from build123d import *

# Parameters (mm, degrees)
SKETCH_1_R           = 14.5
EXTRUDE_1_DEPTH      = 17.3
SKETCH_2_R           = 1.475
EXTRUDE_2_DEPTH      = 8.2
MM_CLEARANCE_1_D     = 3
MM_CLEARANCE_1_DEPTH = 3
MM_CLEARANCE_1_TIP   = 0.901290929
CHAMFER_1_SIZE       = 1
CHAMFER_1_SIZE2      = 3.732050808
FILLET_1_R           = 1
CHAMFER_2_SIZE       = 1
CHAMFER_2_SIZE2      = 3.732050808
MM_CLEARANCE_2_D     = 2
MM_CLEARANCE_2_DEPTH = 3
MM_CLEARANCE_2_TIP   = 0.600860619


with BuildPart() as part:
    # 草图1 → 凸台-拉伸1 (new body)
    with BuildSketch(Plane(origin=(0, 0, 0), x_dir=(1, 0, 0), z_dir=(0, 1, 0))):
        Circle(SKETCH_1_R)
    extrude(amount=EXTRUDE_1_DEPTH)

    # 草图2 → 凸台-拉伸2 (add)
    with BuildSketch(Plane(origin=(0, 17.3, 0), x_dir=(1, 0, 0), z_dir=(0, 1, 0))):
        Circle(SKETCH_2_R)
    extrude(amount=EXTRUDE_2_DEPTH)

    # 大小mm Clearance 暗销槽口1
    with Locations(Plane(origin=(0, 0, 0), x_dir=(-1, 0, 0), z_dir=(0, -1, 0))):
        with Locations((0, -8), (9.5, 0), (0, 8.000635696), (-9.5, 0)):
            Hole(MM_CLEARANCE_1_D / 2, depth=MM_CLEARANCE_1_DEPTH)
            with Locations((0, 0, -(MM_CLEARANCE_1_DEPTH + MM_CLEARANCE_1_TIP / 2))):  # 118° drill point
                Cone(0, MM_CLEARANCE_1_D / 2, MM_CLEARANCE_1_TIP, mode=Mode.SUBTRACT)

    # 倒角1
    chamfer_1_edges = [part.edges().sort_by_distance(p)[0] for p in [
        (-14.5, 0, 0),
    ]]
    chamfer_1_side = [part.faces().sort_by_distance(p)[0] for p in [
        (0, 0, 7.107e-06),
    ]]
    chamfer(chamfer_1_edges, length=CHAMFER_1_SIZE, length2=CHAMFER_1_SIZE2, reference=chamfer_1_side[0])

    # 圆角1
    fillet_1_edges = [part.edges().sort_by_distance(p)[0] for p in [
        (-13.5, 0, 0),
    ]]
    fillet(fillet_1_edges, radius=FILLET_1_R)

    # 倒角2
    chamfer_2_edges = [part.edges().sort_by_distance(p)[0] for p in [
        (-14.5, 17.3, 0),
    ]]
    chamfer_2_side = [part.faces().sort_by_distance(p)[0] for p in [
        (-14.5, 10.516025404, 0),
    ]]
    chamfer(chamfer_2_edges, length=CHAMFER_2_SIZE, length2=CHAMFER_2_SIZE2, reference=chamfer_2_side[0])

    # 大小mm Clearance 暗销槽口2
    with Locations(Plane(origin=(0, 17.3, 0), x_dir=(1, 0, 0), z_dir=(0, 1, 0))):
        with Locations((-4.460030829, 2.575), (4.460030829, 2.575), (0, -5.15)):
            Hole(MM_CLEARANCE_2_D / 2, depth=MM_CLEARANCE_2_DEPTH)
            with Locations((0, 0, -(MM_CLEARANCE_2_DEPTH + MM_CLEARANCE_2_TIP / 2))):  # 118° drill point
                Cone(0, MM_CLEARANCE_2_D / 2, MM_CLEARANCE_2_TIP, mode=Mode.SUBTRACT)


solid = part.part
Work out the finished part from the listing and answer in its coordinate system (mm). A direction names the side the tool comes from. Give positions to 0.01 mm unless a question says otherwise; leave off trailing zeros. Write each loop counter-clockwise with the first axis right and the second up, starting at its lowest first coordinate (ties: lowest second). Pieces come first, ordered by that corner, then holes. Notation, with made-up numbers: M -37.5,84.25 L -29.5,84.25 A6 ccw -29.5,93.25 Z; hole C 55,23 d3. An arc over 180 degrees is marked long. Answer as CSV lines item,"result".
Q1. The mould has two halves that part along X. Classify faces 1 (the cylindrical face through (-1.474, 21.343, -0.065)), 2 (the flat face through (0, 17.3, 2)), 3 (the cylindrical face through (3.506, 15.779, -2.875)), 4 (the cylindrical face through (-11, 2, 0)): +X half, -X half, draft (parallel to the pull), parting line (faces both ways), or undercut.
A:
face 1,"parting line"
face 2,"draft"
face 3,"undercut"
face 4,"undercut"
Q2. A cutting plane is placed at A-A on y = 21. Write down the section's boundary in (x, z) (3 decimals), plus the area to 3 significant figures.
A:
outline,"C 0,0 d2.95"
area,"6.83 mm²"
Q3. A tool of negligible diameter and unlimited length cuts with its end or side. For faces 5 (the cylindrical face through (-0.195, 1.521, -9.488)), 6 (the flat face through (0, 25.5, 0)), 7 (the cylindrical face through (-3.72, 15.78, -3.25)), from which of +Z, -Z, +X, -X, +Y, -Y can it reach the whole face along a straight path? Write none if from no direction.
A:
face 5,"-Y"
face 6,"+Z, -Z, +X, -X, +Y"
face 7,"+Y"
Q4. A cutting plane is placed at B-B on y = 5.5. Write down the section's boundary in (x, z).
A:
outline,"C 0,0 d29"
Q5. Find the intervals of material crossed by probe 1 along Z at (x, y) = (0, 0.8); probe 2 along Y at (x, z) = (-2.75, 5.5); probe 3 along Z at (x, y) = (-4.5, 15.5), in increasing order. Write a range as [from, to].
A:
probe 1,"z = [-13.71, -9.5], [-6.5, 6.5], [9.5, 13.71]"
probe 2,"y = [0, 17.3]"
probe 3,"z = [-13.78, -3.57], [-1.58, 13.78]"
Q6. Given P1, Ø2.5, axis at x = 0, z = -8, coming from the -Y side; P2, Ø1.2, axis at x = 4.46, z = -2.58, coming from the +Y side; P3, Ø8, axis at x = -9.5, y = 15, coming from the +Z side; P4, Ø6, axis at y = 21.5, z = -9.5, coming from the -X side, each flat-ended and moving along its own axis, determine where each tip first touches the part or whether it passes through.
A:
P1,"stops at y = 3.15"
P2,"stops at y = 14.06"
P3,"stops at z = 13.42"
P4,"passes through"
